The drawing under review shows one solid part. Ordinate dimensions are in mm from its lowest x, y, z. Coordinates: 2 decimals unless noted, no trailing zeros. Order: outer loops, then holes, each group sorted by start corner. A loop starts at its lowest first (then second) coordinate and runs counter-clockwise, first axis right, second up. Notation, with made-up numbers: M 65,-25 L 90,-25 A5 ccw 90,-16 Z; hole C -33.5,-5.5 d7. An arc over 180 degrees is marked long. Answer as a JSON object with one key per item and string values.
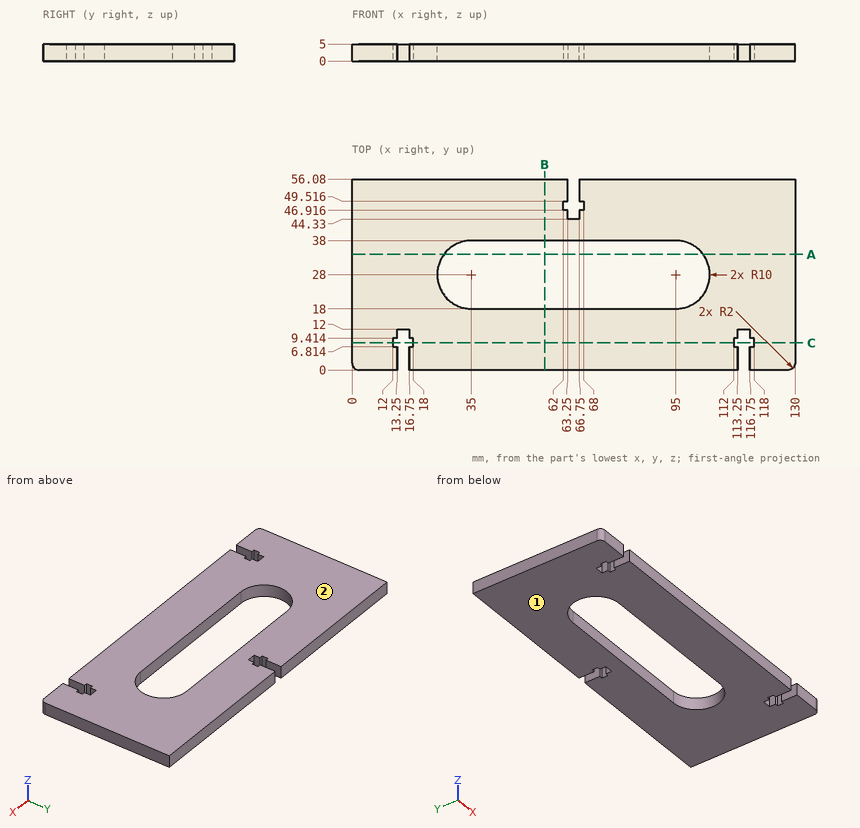
1) Add section A-A (y = 34). State the section outline as (x, z) points, and give its area (3 significant figures).
Taken from the geometry:
{"outline": "M 0,0 L 27,0 L 27,5 L 0,5 Z; M 103,0 L 130,0 L 130,5 L 103,5 Z", "area": "270 mm2"}
2) Mouldability with a two-part tool opening along Z and no side actions: class the marked faces 1 and 2 as released by +Z, released by -Z, zero draft, split by the parting line, or undercut.
Taken from the geometry:
{"face 1": "released by -Z", "face 2": "released by +Z"}
3) To check wall thickness, follow L1, parallel to X at y = 4, z = 3.7; L2, parallel to Y at x = 67.5, z = 4.15; L3, parallel to X at y = 45, z = 0.6. State the ranges of each line that lie inside material, in increasing order.
Taken from the geometry:
{"L1": "x = 0 to 13.25, 16.75 to 113.25, 116.75 to 130", "L2": "y = 0 to 18, 38 to 46.92, 49.52 to 56.08", "L3": "x = 0 to 63.25, 66.75 to 130"}
4) Add section C-C (y = 8). State the section outline as (x, z) points, and give its area (3 significant figures).
Taken from the geometry:
{"outline": "M 0,0 L 12,0 L 12,5 L 0,5 Z; M 18,0 L 112,0 L 112,5 L 18,5 Z; M 118,0 L 130,0 L 130,5 L 118,5 Z", "area": "590 mm2"}
5) Add section B-B (x = 56.5). State the section outline as (y, z) points.
Taken from the geometry:
{"outline": "M 0,0 L 18,0 L 18,5 L 0,5 Z; M 38,0 L 56.08,0 L 56.08,5 L 38,5 Z"}
6) Insertion check: pin 1 Ø1.8 at (x, z) = (64.5, 2) entering from +Y. The pin has a flat end and moves straight along its axis. Give the tip position at first contact, or say it passes through.
Taken from the geometry:
{"pin 1": "stops at y = 44.33"}
